Design review of the part built by this model. Coordinates are the model's own, in mm. A direction names the side the tool comes from. Coordinates: 2 decimals unless noted, no trailing zeros. Write each loop counter-clockwise with the first axis right and the second up, starting at its lowest first coordinate (ties: lowest second). Pieces come first, ordered by that corner, then holes. Notation, with made-up numbers: (0.25, -14.75) -> (17.25, -14.75) arc R26 cw to (17.25, 6.25) -> close; hole circle Ø1 at (66.25, 39.5). An arc over 180 degrees is marked (long way). Answer in a Markdown table with one row per item. Add a question column.
Item 1: Draft analysis for pull direction Z (two halves, no side actions). For faces 1 (the face through (19.493, -4.911, 81.977)), 2 (the face through (-1.6, -9.6, 113)), 3 (the face through (15.43, 9.51, 57.8)), 4 (the face through (0, 9, 2)), state which applies: released by +Z, released by -Z, zero draft, split by the parting line, or undercut.
Item 2: Clearance check with a flat-ended pin moving along its axis: P1, Ø3.5, axis at x = 14.5, z = -92.5, coming from the -Y side. State where the tip first meets the part, or that it passes through.
Item 3: To check wall thickness, follow line 1 (Y direction, x = -3, z = 61); line 2 (X direction, y = -6, z = -81.5); line 3 (Y direction, x = 19.55, z = 84) (3 decimals). State the ranges of each line that lie inside material, in increasing order.
Item 4: Take a section at C-C, the plane z = -74. Write out the cut boundary in (x, y) (3 decimals), and give its area (3 significant figures).
Item 5: Take a section at B-B, the plane y = 0. Write out the cut boundary in (x, z).
Item 6: Take a section at A-A, the plane x = 2. Write out the cut boundary in (y, z), and give its area (3 significant figures).
Item 7: Take a section at D-D, the plane z = 102. Write out the cut boundary in (x, y).
Item 8: For faces 5 (the face through (-15.31, -9.51, -59.66)), 6 (the face through (-13.4, 9.5, -75.7)), list the 3-axis set-ups (+Z, -Z, +X, -X, +Y, -Y) from which the entire face can be reached by the end or side of a thin tool; tool diameter is ignored.
from build123d import *

# Parameters (mm, degrees)
SKETCH_1_W          = 40
SKETCH_1_H          = 20
SKETCH_1_W_2        = 38
SKETCH_1_H_2        = 18
EXTRUDE_1_DEPTH     = 113
SKETCH_2_R          = 6.55
CUT_EXTRUDE_1_DEPTH = 40
SKETCH_3_R          = 2.025
CUT_EXTRUDE_2_DEPTH = 30
SKETCH_4_R          = 2.025
CUT_EXTRUDE_3_DEPTH = 20
SKETCH_6_R          = 2.025
CUT_EXTRUDE_4_DEPTH = 30
SKETCH_9_R          = 3.75
CUT_EXTRUDE_5_DEPTH = 2
SKETCH_10_R         = 2.025
CUT_EXTRUDE_6_DEPTH = 50
SKETCH_11_R         = 3.75
SKETCH_11_R_2       = 2.025
EXTRUDE_2_DEPTH     = 1
SKETCH_13_R         = 2.025
CUT_EXTRUDE_8_DEPTH = 55


with BuildPart() as part:
    # 草图1 → 凸台-拉伸1 (new body, symmetric)
    with BuildSketch(Plane.XY):
        Rectangle(SKETCH_1_W, SKETCH_1_H)
        Rectangle(SKETCH_1_W_2, SKETCH_1_H_2, mode=Mode.SUBTRACT)
    extrude(amount=EXTRUDE_1_DEPTH, both=True)

    # 草图2 → 切除-拉伸1 (cut)
    with BuildSketch(Plane(origin=(20, 0, 0), x_dir=(0, 0, -1), z_dir=(1, 0, 0))):
        with Locations((102, 0)):
            Circle(SKETCH_2_R)
        with Locations((-102, 0)):
            Circle(SKETCH_2_R)
    extrude(amount=-CUT_EXTRUDE_1_DEPTH, mode=Mode.SUBTRACT)

    # 草图3 → 切除-拉伸2 (cut)
    with BuildSketch(Plane(origin=(0, 10, 0), x_dir=(1, 0, 0), z_dir=(0, 1, 0))):
        with Locations((-14.5, 92.5)):
            Circle(SKETCH_3_R)
        with Locations((14.5, 92.5)):
            Circle(SKETCH_3_R)
        with Locations((14.5, -92.5)):
            Circle(SKETCH_3_R)
        with Locations((-14.5, -92.5)):
            Circle(SKETCH_3_R)
    extrude(amount=-CUT_EXTRUDE_2_DEPTH, mode=Mode.SUBTRACT)

    # 草图4 → 切除-拉伸3 (cut)
    with BuildSketch(Plane(origin=(0, 10, 0), x_dir=(1, 0, 0), z_dir=(0, 1, 0))):
        with Locations((-14.5, 74)):
            Circle(SKETCH_4_R)
        with Locations((-14.5, 56)):
            Circle(SKETCH_4_R)
        with Locations((14.5, 56)):
            Circle(SKETCH_4_R)
        with Locations((14.5, 74)):
            Circle(SKETCH_4_R)
        with Locations((14.5, -74)):
            Circle(SKETCH_4_R)
        with Locations((14.5, -56)):
            Circle(SKETCH_4_R)
        with Locations((-14.5, -56)):
            Circle(SKETCH_4_R)
        with Locations((-14.5, -74)):
            Circle(SKETCH_4_R)
    extrude(amount=-CUT_EXTRUDE_3_DEPTH, mode=Mode.SUBTRACT)

    # 草图6 → 切除-拉伸4 (cut)
    with BuildSketch(Plane(origin=(0, 10, 0), x_dir=(1, 0, 0), z_dir=(0, 1, 0))):
        with Locations((-14.5, 42)):
            Circle(SKETCH_6_R)
        with Locations((14.5, 42)):
            Circle(SKETCH_6_R)
        with Locations((-14.5, -42)):
            Circle(SKETCH_6_R)
        with Locations((14.5, -42)):
            Circle(SKETCH_6_R)
    extrude(amount=-CUT_EXTRUDE_4_DEPTH, mode=Mode.SUBTRACT)

    # 草图9 → 切除-拉伸5 (cut)
    with BuildSketch(Plane.XZ.offset(10)):
        with Locations((-14.5, 74)):
            Circle(SKETCH_9_R)
        with Locations((14.5, 74)):
            Circle(SKETCH_9_R)
        with Locations((-14.5, 56)):
            Circle(SKETCH_9_R)
        with Locations((-14.5, 42)):
            Circle(SKETCH_9_R)
        with Locations((14.5, 42)):
            Circle(SKETCH_9_R)
        with Locations((14.5, 56)):
            Circle(SKETCH_9_R)
        with Locations((14.5, -56)):
            Circle(SKETCH_9_R)
        with Locations((14.5, -42)):
            Circle(SKETCH_9_R)
        with Locations((-14.5, -42)):
            Circle(SKETCH_9_R)
        with Locations((-14.5, -56)):
            Circle(SKETCH_9_R)
        with Locations((14.5, -74)):
            Circle(SKETCH_9_R)
        with Locations((-14.5, -74)):
            Circle(SKETCH_9_R)
    extrude(amount=-CUT_EXTRUDE_5_DEPTH, mode=Mode.SUBTRACT)

    # 草图10 → 切除-拉伸6 (cut)
    with BuildSketch(Plane.ZY.offset(20)):
        with Locations((84, 5)):
            Circle(SKETCH_10_R)
        with Locations((84, -5)):
            Circle(SKETCH_10_R)
        with Locations((-84, 5)):
            Circle(SKETCH_10_R)
        with Locations((-84, -5)):
            Circle(SKETCH_10_R)
    extrude(amount=-CUT_EXTRUDE_6_DEPTH, mode=Mode.SUBTRACT)

    # 草图11 → 凸台-拉伸2 (add)
    with BuildSketch(Plane.XZ.offset(10)):
        with Locations((14.5, -74)):
            Circle(SKETCH_11_R)
        with Locations((14.5, -74)):
            Circle(SKETCH_11_R_2, mode=Mode.SUBTRACT)
        with Locations((-14.5, -74)):
            Circle(SKETCH_11_R)
        with Locations((-14.5, -74)):
            Circle(SKETCH_11_R_2, mode=Mode.SUBTRACT)
        with Locations((-14.5, 74)):
            Circle(SKETCH_11_R)
        with Locations((-14.5, 74)):
            Circle(SKETCH_11_R_2, mode=Mode.SUBTRACT)
        with Locations((14.5, 74)):
            Circle(SKETCH_11_R)
        with Locations((14.5, 74)):
            Circle(SKETCH_11_R_2, mode=Mode.SUBTRACT)
    extrude(amount=-EXTRUDE_2_DEPTH)

    # 草图13 → 切除-拉伸8 (cut)
    with BuildSketch(Plane(origin=(20, 0, 0), x_dir=(0, 0, -1), z_dir=(1, 0, 0))):
        with Locations((-69, 5)):
            Circle(SKETCH_13_R)
        with Locations((-69, -5)):
            Circle(SKETCH_13_R)
        with Locations((69, -5)):
            Circle(SKETCH_13_R)
        with Locations((69, 5)):
            Circle(SKETCH_13_R)
    extrude(amount=-CUT_EXTRUDE_8_DEPTH, mode=Mode.SUBTRACT)


solid = part.part
Answers:
| question | item | result |
|---|---|---|
| 1 | face 1 | undercut |
| 1 | face 2 | released by +Z |
| 1 | face 3 | undercut |
| 1 | face 4 | zero draft |
| 2 | P1 | passes through |
| 3 | line 1 | y = -10 to -9, 9 to 10 |
| 3 | line 2 | x = -20 to -19, 19 to 20 |
| 3 | line 3 | y = -10 to -7.025, -2.975 to 2.975, 7.025 to 10 |
| 4 | outline | (-20, -10) -> (-16.525, -10) -> (-16.525, -9) -> (-19, -9) -> (-19, 9) -> (-16.525, 9) -> (-16.525, 10) -> (-20, 10) -> close; (-12.475, -10) -> (12.475, -10) -> (12.475, -9) -> (-12.475, -9) -> close; (-12.475, 9) -> (12.475, 9) -> (12.475, 10) -> (-12.475, 10) -> close; (16.525, -10) -> (20, -10) -> (20, 10) -> (16.525, 10) -> (16.525, 9) -> (19, 9) -> (19, -9) -> (16.525, -9) -> close |
| 4 | area | 99.8 mm^2 |
| 5 | outline | (-20, -113) -> (-19, -113) -> (-19, -108.55) -> (-20, -108.55) -> close; (-20, -95.45) -> (-19, -95.45) -> (-19, 95.45) -> (-20, 95.45) -> close; (-20, 108.55) -> (-19, 108.55) -> (-19, 113) -> (-20, 113) -> close; (19, -113) -> (20, -113) -> (20, -108.55) -> (19, -108.55) -> close; (19, -95.45) -> (20, -95.45) -> (20, 95.45) -> (19, 95.45) -> close; (19, 108.55) -> (20, 108.55) -> (20, 113) -> (19, 113) -> close |
| 6 | outline | (-10, -113) -> (-9, -113) -> (-9, 113) -> (-10, 113) -> close; (9, -113) -> (10, -113) -> (10, 113) -> (9, 113) -> close |
| 6 | area | 452 mm^2 |
| 7 | outline | (-20, -10) -> (20, -10) -> (20, -6.55) -> (19, -6.55) -> (19, -9) -> (-19, -9) -> (-19, -6.55) -> (-20, -6.55) -> close; (-20, 6.55) -> (-19, 6.55) -> (-19, 9) -> (19, 9) -> (19, 6.55) -> (20, 6.55) -> (20, 10) -> (-20, 10) -> close |
| 8 | face 5 | -Y |
| 8 | face 6 | +Y, -Y |
